Input: part model. Units: mm. Frame: model coordinates. A direction names the side the tool comes from. Coordinates: 2 decimals unless noted, no trailing zeros. Loops run counter-clockwise (first coordinate to the right, second up) from the corner with the lowest first, then second, coordinate; pieces in that order, holes last.
```python
from build123d import *

# Parameters (mm, degrees)
SKETCH1_W           = 101.6
SKETCH1_H           = 76.2
BOSS_EXTRUDE1_DEPTH = 25.4
SKETCH2_W           = 31.75
SKETCH2_H           = 19.304
CUT_EXTRUDE2_DEPTH  = 26.4
SKETCH4_R           = 6.35
CUT_EXTRUDE3_DEPTH  = 57.896


with BuildPart() as part:
    # Sketch1 → Boss-Extrude1 (new body)
    with BuildSketch(Plane(origin=(0, 0, 0), x_dir=(1, 0, 0), z_dir=(0, 1, 0))):
        Rectangle(SKETCH1_W, SKETCH1_H)
    extrude(amount=BOSS_EXTRUDE1_DEPTH)

    # Sketch2 → Cut-Extrude2 (cut, through all)
    with BuildSketch(Plane(origin=(0, 25.4, 0), x_dir=(1, 0, 0), z_dir=(0, 1, 0))):
        with Locations((-34.925, 28.448)):
            Rectangle(SKETCH2_W, SKETCH2_H)
        with Locations((-34.925, -28.448)):
            Rectangle(SKETCH2_W, SKETCH2_H)
    extrude(amount=-CUT_EXTRUDE2_DEPTH, mode=Mode.SUBTRACT)

    # Sketch4 → Cut-Extrude3 (cut, through all)
    with BuildSketch(Plane.XY.offset(18.796)):
        with Locations((-34.925, 12.7)):
            Circle(SKETCH4_R)
    extrude(amount=-CUT_EXTRUDE3_DEPTH, mode=Mode.SUBTRACT)


solid = part.part
```
Item 1: Contact query for flat-ended pins moving along their axis: P1, Ø10, axis at x = -30, y = 14.5, coming from the -Z side; P2, Ø6, axis at y = 17.5, z = 25, coming from the -X side. Output: stop coordinate, or through.
Result:
P1: stops at z = -18.8
P2: stops at x = -19.05
Item 2: Section query B-B (y = 4.25). Output: boundary loops of the cut face in (x, z), then the cut area to 3 significant figures.
Result:
outline: (-50.8, -18.8) - (-19.05, -18.8) - (-19.05, -38.1) - (50.8, -38.1) - (50.8, 38.1) - (-19.05, 38.1) - (-19.05, 18.8) - (-50.8, 18.8) - close
area: 6,520 mm2
Item 3: Section query D-D (z = 5.5). Output: boundary loops of the cut face in (x, y) (3 decimals), then the cut area to 3 significant figures.
Result:
outline: (-50.8, 0) - (50.8, 0) - (50.8, 25.4) - (-50.8, 25.4) - close; hole circle Ø12.7 at (-34.925, 12.7)
area: 2,450 mm2
Item 4: Section query C-C (x = -40). Output: boundary loops of the cut face in (y, z), then the cut area to 3 significant figures.
Result:
outline: (0, -18.8) - (8.88, -18.8) - (8.88, 18.8) - (0, 18.8) - close; (16.52, -18.8) - (25.4, -18.8) - (25.4, 18.8) - (16.52, 18.8) - close
area: 668 mm2
Item 5: Mould query, pull axis Y, two halves, no side actions, for faces 4 (the face through (-19.05, 13, 29)), 5 (the face through (-39.6, 17, 0.3)), 6 (the face through (11, 25.4, -1)). Classes: +Y half, -Y half, draft (parallel to the pull), parting line (faces both ways), or undercut.
Result:
face 4: draft
face 5: undercut
face 6: +Y half
Item 6: Line query: L1, parallel to Z at x = -20, y = 8.5; L2, parallel to X at y = 18, z = -12; L3, parallel to X at y = 12.75, z = -1. Output: solid intervals per line, ascending.
Result:
L1: z = -18.8 to 18.8
L2: x = -50.8 to -38.42, -31.43 to 50.8
L3: x = -50.8 to -41.27, -28.58 to 50.8
Item 7: Reachability of faces 1 (the face through (-32, 19, 18.796)), 2 (the face through (-19.05, 13, -28)), 3 (the face through (15, 13, -38.1)) from +Z, -Z, +X, -X, +Y, -Y: full face, straight path, thin tool, end or side. Return the list, or none.
Result:
face 1: +Z, -X, +Y, -Y
face 2: -Z, -X, +Y, -Y
face 3: -Z, +X, -X, +Y, -Y
Item 8: Section query A-A (y = 12.7). Output: boundary loops of the cut face in (x, z) (3 decimals).
Result:
outline: (-50.8, -18.796) - (-41.275, -18.796) - (-41.275, 18.796) - (-50.8, 18.796) - close; (-28.575, -18.796) - (-19.05, -18.796) - (-19.05, -38.1) - (50.8, -38.1) - (50.8, 38.1) - (-19.05, 38.1) - (-19.05, 18.796) - (-28.575, 18.796) - close
